Autodesk Inventor part; units mm, degrees
ref_plane "Work Plane1" through (-20.5, 0, -41) normal (1, 0, 0) x (0, 0, -1)
ref_plane "YZ Plane" through (0, 0, 0) normal (1, 0, 0) x (0, 1, 0)
ref_plane "XZ Plane" through (0, 0, 0) normal (0, 1, 0) x (-1, 0, 0)
sketch "Sketch1" plane through (0, 0, 0) normal (0, 1, 0) x (-1, 0, 0)
  line L0 (0, 0) -> (41, 0)
  line L1 (41, 0) -> (41, -41)
  line L2 (41, -41) -> (0, -41)
  line L3 (0, -41) -> (0, 0)
  dimension "d0" = 41
  dimension "d1" = 41
extrude "Extrusion1" add sketch "Sketch1" along normal blind 9.5
sketch "Sketch3" plane through (0, 9.5, 0) normal (0, 1, 0) x (1, 0, 0)
  circle A0 centre (-20.5, 20.5) radius 10
  point P0 (0, 0)
  dimension "d5" = 20
extrude "Extrusion2" cut sketch "Sketch3" against normal blind 10
sketch "Sketch4" plane through (0, 9.5, 0) normal (0, 1, 0) x (1, 0, 0)
  circle A0 centre (-20.5, 20.5) radius 10
  circle A1 centre (-20.5, 20.5) radius 11.75
  point P0 (0, 0)
  dimension "d8" = 23.5
extrude "Extrusion3" cut sketch "Sketch4" against normal blind 5
sketch "Sketch5" plane through (0, 9.5, 0) normal (0, 1, 0) x (1, 0, 0)
  line L0 (-41, 41) -> (-41, 0)
  line L1 (-41, 0) -> (0, 0)
  line L2 (0, 0) -> (0, 41)
  line L3 (0, 41) -> (-41, 41)
  line L4 (-41, 41) -> (-41, 0)
  circle A0 centre (-20.5, 20.5) radius 11.75
  circle A1 centre (-20.5, 20.5) radius 10
extrude "Extrusion4" add sketch "Sketch5" along normal blind 4.5 contours L3 L2 L1 L0 | A0
sketch "Sketch6" plane through (-41, 0, 0) normal (0, 0, 1) x (1, 0, 0)
  line L0 (0, 0) -> (0, 14)
  line L1 (0, 14) -> (41, 14)
  line L2 (41, 14) -> (41, 0)
  line L3 (41, 0) -> (0, 0)
  line L4 (0, 0) -> (0, 14)
extrude "Extrusion5" cut sketch "Sketch6" against normal blind 20.5
sketch "Sketch8" plane through (-41, 0, -20.5) normal (0, 0, 1) x (1, 0, 0)
  circle A0 centre (4, 10) radius 1.8
  point P0 (41, 0)
  dimension "d15" = 3.6
extrude "Extrusion6" cut sketch "Sketch8" against normal blind 20.5
ref_plane "Work Plane1" through (-20.5, 0, -41) normal (1, 0, 0) x (0, 0, -1)
mirror "Mirror1" about plane through (-20.5, 0, -41) normal (1, 0, 0) of "Extrusion6"
sketch "Sketch9" plane through (-41, 0, -20.5) normal (0, 0, 1) x (1, 0, 0)
  line L0 (10.5, 14) -> (10.5, 9.5)
  line L1 (8.75, 4.5) -> (10.5, 4.5)
  line L2 (10.5, 9.5) -> (8.75, 9.5)
  line L3 (8.75, 9.5) -> (8.75, 4.5)
  line L4 (8.75, 4.5) -> (10.5, 4.5)
  line L5 (10.5, 4.5) -> (10.5, 9.5)
  point P0 (41, 0)
sketch "Sketch11" plane through (0, 4.5, 0) normal (0, 1, 0) x (1, 0, 0)
  arc A0 (-10.5, 20.5) -> (-30.5, 20.5) centre (-20.5, 20.5) ccw
  arc A1 (-9.625, 20.5) -> (-31.375, 20.5) centre (-20.5, 20.5) ccw
  line L0 (-41, 41) -> (-41, 20.5)
  point P0 (0, 0)
sweep "Sweep1" add profiles "Sketch9" path "Sketch11" path curves A1
sketch "Sketch12" plane through (-41, 0, -20.5) normal (0, 0, 1) x (1, 0, 0)
  line L0 (10.5, 14) -> (10.5, 0)
  circle A0 centre (10.5, 7) radius 0.8
  point P0 (41, 0)
  dimension "d21" = 1.6
sketch3d "3D Sketch1"
  arc A0 (-30.5, 14, -20.5) -> (-27.5711, 14, -27.5711) centre (-20.5, 14, -20.5) ccw
  arc A1 (-27.5711, 14, -27.5711) -> (-20.5, 14, -30.5) centre (-20.5, 14, -20.5) ccw
  arc A2 (-20.5, 14, -30.5) -> (-13.4289, 14, -27.5711) centre (-20.5, 14, -20.5) ccw
  arc A3 (-13.4289, 14, -27.5711) -> (-10.5, 14, -20.5) centre (-20.5, 14, -20.5) ccw
sweep "Sweep2" cut profiles "Sketch12" path "3D Sketch1"
sketch "Sketch13" plane through (0, 0, 0) normal (0, -1, 0) x (1, 0, 0)
  line L0 (-53.975, -9.525) -> (46.0375, -9.525)
  line L1 (46.0375, -9.525) -> (46.0375, -71.4375)
  line L2 (46.0375, -71.4375) -> (-53.975, -71.4375)
  line L3 (-53.975, -71.4375) -> (-53.975, -9.525)
  point P0 (0, 0)
extrude "Extrusion7" cut sketch "Sketch13" against normal blind 2
sketch "Sketch14" plane through (-41, 0, -20.5) normal (0, 0, 1) x (1, 0, 0)
  line L0 (-1.5875, 15.875) -> (46.0375, 15.875)
  line L1 (46.0375, 15.875) -> (46.0375, -1.5875)
  line L2 (46.0375, -1.5875) -> (-1.5875, -1.5875)
  line L3 (-1.5875, -1.5875) -> (-1.5875, 15.875)
  point P0 (41, 0)
extrude "Extrusion8" cut sketch "Sketch14" against normal blind 0.7
sketch "Sketch15" plane through (0, 14, 0) normal (0, 1, 0) x (1, 0, 0)
  arc A0 (-10.5245, 21.2) -> (-30.4755, 21.2) centre (-20.5, 20.5) ccw
  circle A1 centre (-20.5, 20.5) radius 10.9575
  point P0 (0, 0)
  dimension "d28" = 21.915
extrude "Extrusion9" cut sketch "Sketch15" against normal blind 15
sketch "Sketch16" plane through (-41, 0, -21.2) normal (0, 0, 1) x (1, 0, 0)
  line L0 (9.5649, 2) -> (9.5649, 14)
  circle A0 centre (9.5649, 7) radius 0.8
  point P0 (41, 0)
  dimension "d31" = 1.6
sketch "Sketch17" plane through (0, 14, 0) normal (0, 1, 0) x (1, 0, 0)
  arc A0 (-9.5649, 21.2) -> (-31.4351, 21.2) centre (-20.5, 20.5) ccw
  arc A1 (-7.5073, 21.2) -> (-33.4927, 21.2) centre (-20.5, 20.5) ccw
  point P0 (0, 0)
sketch3d "3D Sketch2"
  arc A0 (-31.4351, 14, -21.2) -> (-9.5649, 14, -21.2) centre (-20.5, 14, -20.5) ccw
sweep "Sweep3" cut profiles "Sketch16" path "3D Sketch2"
sketch "Sketch18" plane through (-41, 0, -21.2) normal (0, 0, 1) x (1, 0, 0)
  line L0 (31.4351, 7.8) -> (31.4351, 6.2)
  circle A0 centre (31.4351, 7) radius 0.8
  point P0 (41, 0)
sketch3d "3D Sketch3"
  arc A0 (-9.5649, 14, -21.2) -> (-31.4351, 14, -21.2) centre (-20.5, 14, -20.5) ccw
sweep "Sweep4" cut profiles "Sketch18" path "3D Sketch3"
sketch "Sketch19" plane through (-41, 0, -21.2) normal (0, 0, 1) x (1, 0, 0)
  line L0 (0, 2) -> (0, 14)
  line L1 (41, 2) -> (41, 14)
  line L2 (0, 14) -> (41, 14)
  line L3 (41, 14) -> (41, 2)
  line L4 (41, 2) -> (0, 2)
  line L5 (0, 2) -> (0, 14)
  point P0 (41, 0)
extrude "Extrusion10" cut sketch "Sketch19" against normal blind 0.3
sketch "Sketch20" plane through (-41, 0, -21.5) normal (0, 0, 1) x (1, 0, 0)
  line L0 (9.5882, 6.2) -> (9.5882, 2)
  line L1 (9.5882, 2) -> (10.5882, 2)
  line L2 (10.5882, 2) -> (10.5882, 5)
  line L3 (10.5882, 5) -> (9.5882, 5)
  line L4 (9.5882, 5) -> (9.5882, 2)
  point P0 (41, 0)
  dimension "d38" = 1
  dimension "d39" = 3
sweep "Sweep5" add profiles "Sketch20" path "Sketch17" path curves A0
sketch "Sketch21" plane through (-41, 0, -21.5) normal (0, 0, 1) x (1, 0, 0)
  line L0 (0, 2) -> (0, 14)
  line L1 (41, 2) -> (0, 2)
  line L2 (0, 14) -> (41, 14)
  line L3 (41, 14) -> (41, 2)
  line L4 (41, 2) -> (0, 2)
  line L5 (0, 2) -> (0, 14)
  point P0 (41, 0)
extrude "Extrusion11" cut sketch "Sketch21" along normal blind 10
chamfer "Chamfer1" distance 1 angle 45 2 edges at (-8.7866, 7, -21.5) (-32.2134, 7, -21.5)
chamfer "Chamfer2" distance 0.3 angle 45 2 edges at (-20.4996, 7.8, -31.4575) (-20.4997, 6.2, -31.4575)
properties part number "7 peristaltic pump lid with lip2"
Build history of the part. All positions in model axes, mm. A direction names the side the tool comes from. Give positions to 0.01 mm unless a question says otherwise; leave off trailing zeros. Loops run counter-clockwise (first coordinate to the right, second up) from the corner with the lowest first, then second, coordinate; pieces in that order, holes last.
1) Two-plate mould, pull along X, no slides. Class faces 1 (the face through (-41, 8, -31)), 2 (the face through (0, 8, -31)), 3 (the face through (-20, 2, -33)), 4 (the face through (-36.169, 8.403, -31.114)): released by +X, released by -X, zero draft, split by the parting line, or undercut.
Values follow:
face 1: released by -X
face 2: released by +X
face 3: zero draft
face 4: undercut
2) Probe line 1 along Y through (x, z) = (-37, -30.25); line 2 along X through (y, z) = (9.75, -27.75); line 3 along X through (y, z) = (11.25, -25). List the from-to ranges inside material, lowest first.
Values follow:
line 1: y = 2 to 8.2, 11.8 to 14
line 2: x = -41 to -38.78, -35.22 to -28.72, -12.28 to -5.78, -2.22 to 0
line 3: x = -41 to -38.3, -35.7 to -30.49, -10.51 to -5.3, -2.7 to 0
3) Band-saw the part on B-B on x = -37. List the corners of the cut face in (y, z).
Values follow:
outline: (2, -41) - (8.2, -41) - (8.2, -21.5) - (2, -21.5) - close; (11.8, -41) - (14, -41) - (14, -21.5) - (11.8, -21.5) - close
4) 3-axis set-ups, long thin cutter, end or side, ignore diameter. For faces 5 (the face through (-21, 8, -41)), 6 (the face through (-20, 5, -31)): which of +Z, -Z, +X, -X, +Y, -Y reach the whole face in a straight line?
Values follow:
face 5: -Z, +X, -X, +Y, -Y
face 6: +Z, +Y
5) Band-saw the part on A-A on y = 10. List the corners of the cut face in (x, z) (1 decimal), then the cut area to 3 significant figures.
Values follow:
outline: (-41, -41) - (-38.8, -41) - (-38.8, -21.5) - (-41, -21.5) - close; (-35.2, -41) - (-5.8, -41) - (-5.8, -21.5) - (-9.6, -21.5) arc R11 cw to (-31.4, -21.5) - (-35.2, -21.5) - close; (-2.2, -41) - (0, -41) - (0, -21.5) - (-2.2, -21.5) - close
area: 492 mm2
6) Band-saw the part on C-C on z = -33.5. List the corners of the cut face in (x, y).
Values follow:
outline: (-41, 2) - (0, 2) - (0, 14) - (-41, 14) - close; hole circle Ø3.6 at (-37, 10); hole circle Ø3.6 at (-4, 10)
7) Band-saw the part on D-D on z = -24. State how many separate pieces and enclosed holes the cut face has, then the cut area to 3 significant figures.
Values follow:
separate pieces: 2
enclosed holes: 2
area: 226 mm2
